Autodesk Inventor part; units mm, degrees
ref_plane "YZ Plane" through (0, 0, 0) normal (1, 0, 0) x (0, 1, 0)
ref_plane "XZ Plane" through (0, 0, 0) normal (0, 1, 0) x (-1, 0, 0)
ref_plane "XY Plane" through (0, 0, 0) normal (0, 0, 1) x (1, 0, 0)
sketch "Sketch1" plane through (0, 0, 0) normal (0, 1, 0) x (-1, 0, 0)
  circle A0 centre (0, 0) radius 190.5
  dimension "d0" = 381
extrude "Extrusion1" add sketch "Sketch1" along normal blind 25.4
sketch "Sketch2" plane through (0, 25.4, 0) normal (0, 1, 0) x (1, 0, 0)
  circle A0 centre (0, 0) radius 177.8
  circle A1 centre (0, 0) radius 190.5
  dimension "d3" = 355.6
extrude "Extrusion2" add sketch "Sketch2" along normal blind 558.8
sketch "Sketch3" plane through (0, 584.2, 0) normal (0, 1, 0) x (1, 0, 0)
  circle A0 centre (0, 0) radius 190.8969
  dimension "d6" = 381.7937
extrude "Extrusion3" add sketch "Sketch3" along normal blind 50.8
ref_plane "Work Plane2" through (190.5, 0, 0) normal (1, 0, 0) x (0, 1, 0)
ref_plane "Work Plane1" through (228.6, -12.7, -4375.1201) normal (1, 0, 0) x (0, 1, 0)
ref_plane "Work Plane4" through (0, 0, 190.5) normal (0, 0, 1) x (1, 0, 0)
ref_plane "Work Plane3" through (-228.6, -12.7, 203.2) normal (0, 0, 1) x (1, 0, 0)
properties part number "Tun-Placeholder"
Design review of the part built by this model. Coordinates are the model's own, in mm. A direction names the side the tool comes from. Coordinates: 2 decimals unless noted, no trailing zeros. Order: outer loops, then holes, each group sorted by start corner. A loop starts at its lowest first (then second) coordinate and runs counter-clockwise, first axis right, second up. Notation, with made-up numbers: (15.25, -37) - (49.25, -37) arc R36 ccw to (49.25, -2) - close; hole circle Ø1 at (19, -4). An arc over 180 degrees is marked (long way). Put each result on its own line as item: value.
1) Tool access review of faces 1 (the face through (-140.699, 609.244, 129.017)), 2 (the face through (-2, 584.2, -2)): name each direction out of +Z, -Z, +X, -X, +Y, -Y from which nothing blocks a thin tool from reaching the whole face with its end or side.
Response values:
face 1: +Y, -Y
face 2: none
2) Wall thickness on L1, parallel to Z at x = 0, y = 242; L2, parallel to Y at x = 1, z = -7: over which ranges is each line inside the solid? List them lowest first. Write a range as from..to.
Response values:
L1: z = -190.5..-177.8, 177.8..190.5
L2: y = 0..25.4, 584.2..635
3) Take a section at A-A, the plane z = -10. Give the boundary of the cut face in (x, y).
Response values:
outline: (-190.63, 584.2) - (-190.24, 584.2) - (-190.24, 0) - (190.24, 0) - (190.24, 584.2) - (190.63, 584.2) - (190.63, 635) - (-190.63, 635) - close; hole (-177.52, 25.4) - (177.52, 25.4) - (177.52, 584.2) - (-177.52, 584.2) - close
4) Take a section at B-B, the plane y = 541. Give the boundary of the cut face in (x, z), and give its area (3 significant figures).
Response values:
outline: circle Ø381 at (0, 0); hole circle Ø355.6 at (0, 0)
area: 14,700 mm²
5) The part is to be moulded in two halves that separate along Y. For faces 3 (the face through (-3, 635, -3)), 4 (the face through (169.59, 300.89, 53.41)), 5 (the face through (3, 0, 3)), say which applies: released by +Y, released by -Y, zero draft, split by the parting line, or undercut.
Response values:
face 3: released by +Y
face 4: undercut
face 5: released by -Y
6) Insertion check: P1, Ø5, axis at y = 345, z = -94, coming from the +X side; P2, Ø3, axis at y = 144, z = 150.5, coming from the +X side; P3, Ø1, axis at x = -77.5, y = 520.5, coming from the +Z side. Each pin has a flat end and moves straight along its axis. Give the tip position at first contact, or say it passes through.
Response values:
P1: stops at x = 167.09
P2: stops at x = 118.7
P3: stops at z = 174.24
7) Take a section at C-C, the plane z = -124. Give the boundary of the cut face in (x, y).
Response values:
outline: (-145.14, 584.2) - (-144.62, 584.2) - (-144.62, 0) - (144.62, 0) - (144.62, 584.2) - (145.14, 584.2) - (145.14, 635) - (-145.14, 635) - close; hole (-127.42, 25.4) - (127.42, 25.4) - (127.42, 584.2) - (-127.42, 584.2) - close
